```python
from build123d import *

# Parameters (mm, degrees)
SKETCH1_W           = 20
SKETCH1_H           = 20
BOSS_EXTRUDE1_DEPTH = 2
SKETCH2_W           = 20
SKETCH2_H           = 2
BOSS_EXTRUDE2_DEPTH = 16
SKETCH3_R           = 2.5
CUT_EXTRUDE1_DEPTH  = 22.354156504
SKETCH4_R           = 2.5
CUT_EXTRUDE2_DEPTH  = 28.349588662


with BuildPart() as part:
    # Sketch1 → Boss-Extrude1 (new body)
    with BuildSketch(Plane(origin=(0, 0, 0), x_dir=(1, 0, 0), z_dir=(0, 1, 0))):
        Rectangle(SKETCH1_W, SKETCH1_H)
    extrude(amount=BOSS_EXTRUDE1_DEPTH)

    # Sketch2 → Boss-Extrude2 (add)
    with BuildSketch(Plane(origin=(0, 2, 0), x_dir=(1, 0, 0), z_dir=(0, 1, 0))):
        with Locations((0, 9)):
            Rectangle(SKETCH2_W, SKETCH2_H)
    extrude(amount=BOSS_EXTRUDE2_DEPTH)

    # Sketch3 → Cut-Extrude1 (cut, through all)
    with BuildSketch(Plane(origin=(0, 2, 0), x_dir=(1, 0, 0), z_dir=(0, 1, 0))):
        with Locations(Location((0, -1, 0), (0, 0, 270))):
            Circle(SKETCH3_R)
    extrude(amount=-CUT_EXTRUDE1_DEPTH, mode=Mode.SUBTRACT)

    # Sketch4 → Cut-Extrude2 (cut, through all)
    with BuildSketch(Plane.XY.offset(-8)):
        with Locations((0, 10)):
            Circle(SKETCH4_R)
    extrude(amount=-CUT_EXTRUDE2_DEPTH, mode=Mode.SUBTRACT)


solid = part.part
```
Check sheet for the modelled part. Datum: model origin and axes. Units: mm. A direction names the side the tool comes from. Round coordinates to 2 decimals unless told otherwise and drop trailing zeros. Loops run counter-clockwise (first coordinate to the right, second up) from the corner with the lowest first, then second, coordinate; pieces in that order, holes last. Notation, with made-up numbers: (37.5, 53.25) - (69.5, 53.25) arc R33 ccw to (69.5, 92.25) - close; hole circle Ø8 at (55, 81). An arc over 180 degrees is marked (long way). Answer as a JSON object with one key per item and string values. Group by question number.
Q1. Mould release check, pull along Z, two halves, no side actions. Record for faces 3 (the face through (-2, 8, -8)), 4 (the face through (0, 18, -9)), 5 (the face through (0.751, 1.014, 3.385)): released by +Z, released by -Z, zero draft, split by the parting line, or undercut.
Q2. Sectioned sample at B-B, the plane x = 0. Enter the section's corners in (y, z), plus the area to 3 significant figures.
Q3. Gauge pin test, flat ends, axial feed: P1, Ø9, axis at x = -2, z = -2, coming from the +Y side; P2, Ø1, axis at x = 5.5, y = 10.5, coming from the +Z side; P3, Ø3, axis at x = 0, y = 10, coming from the +Z side. Record the tip position at first contact, or that the pin passes through.
Q4. Sectioned sample at C-C, the plane z = 1. Enter the section's corners in (x, y).
Q5. Set-up check for faces 1 (the face through (0, 7, -10)), 2 (the face through (-2, 2, -1)): record each of +Z, -Z, +X, -X, +Y, -Y from which the full face is reachable in a straight line by a thin tool's end or side.
Q6. Sectioned sample at D-D, the plane x = 7. Enter the section's corners in (y, z).
Q7. Scan lines: line 1 along X through (y, z) = (1.5, 1); line 2 along Z through (x, y) = (-0.5, 3.5); line 3 along Y through (x, z) = (0, -9.2). Record each from-to range of solid material in increasing order. Write a range as [from, to].
Q8. Sectioned sample at A-A, the plane y = 10. Enter the section's corners in (x, z).
Solution:
{
 "1": {"face 3": "released by +Z", "face 4": "zero draft", "face 5": "undercut"},
 "2": {"outline": "(0, -10) - (7.5, -10) - (7.5, -8) - (2, -8) - (2, -1.5) - (0, -1.5) - close; (0, 3.5) - (2, 3.5) - (2, 10) - (0, 10) - close; (12.5, -10) - (18, -10) - (18, -8) - (12.5, -8) - close", "area": "52.0 mm²"},
 "3": {"P1": "stops at y = 2", "P2": "stops at z = -8", "P3": "passes through"},
 "4": {"outline": "(-10, 0) - (-2.5, 0) - (-2.5, 2) - (-10, 2) - close; (2.5, 0) - (10, 0) - (10, 2) - (2.5, 2) - close"},
 "5": {"face 1": "-Z, +X, -X, +Y, -Y", "face 2": "+Z, +X, -X, +Y"},
 "6": {"outline": "(0, -10) - (18, -10) - (18, -8) - (2, -8) - (2, 10) - (0, 10) - close"},
 "7": {"line 1": "x = [-10, -2.5], [2.5, 10]", "line 2": "z = [-10, -8]", "line 3": "y = [0, 7.5], [12.5, 18]"},
 "8": {"outline": "(-10, -10) - (-2.5, -10) - (-2.5, -8) - (-10, -8) - close; (2.5, -10) - (10, -10) - (10, -8) - (2.5, -8) - close"}
}
